Autodesk Inventor part; units mm, degrees
ref_plane "YZ Plane" through (0, 0, 0) normal (1, 0, 0) x (0, 1, 0)
ref_plane "XZ Plane" through (0, 0, 0) normal (0, 1, 0) x (-1, 0, 0)
ref_plane "XY Plane" through (0, 0, 0) normal (0, 0, 1) x (1, 0, 0)
sketch "Sketch1" plane through (0, 0, 0) normal (0, 1, 0) x (-1, 0, 0)
  line L0 (55, -86.5) -> (-55, -86.5)
  line L1 (-55, -86.5) -> (-55, 86.5)
  line L2 (-55, 86.5) -> (55, 86.5)
  line L3 (55, 86.5) -> (55, -86.5)
  line L4 (55, -86.5) -> (-55, 86.5) construction
  line L5 (-55, -86.5) -> (55, 86.5) construction
  point P0 (0, 0)
  dimension "d0" = 110
  dimension "d1" = 173
extrude "Extrusion1" add sketch "Sketch1" along normal blind 5
sketch "Sketch2" plane through (0, 5, 0) normal (0, 1, 0) x (1, 0, 0)
  line L0 (-55, -86.5) -> (55, -86.5)
  line L1 (-55, -86.5) -> (-60, -86.5)
  line L2 (-60, -86.5) -> (-60, 86.5)
  line L3 (-60, 86.5) -> (-55, 86.5)
  line L4 (-55, 86.5) -> (-55, -86.5)
  point P0 (0, 0)
  dimension "d4" = 5
extrude "Extrusion2" add sketch "Sketch2" against normal blind 34.5
sketch "Sketch3" plane through (0, 5, 0) normal (0, 1, 0) x (1, 0, 0)
  line L0 (55, -86.5) -> (55, 86.5)
  line L1 (55, -86.5) -> (60, -86.5)
  line L2 (60, -86.5) -> (60, 86.5)
  line L3 (60, 86.5) -> (55, 86.5)
  line L4 (55, 86.5) -> (55, -86.5)
  point P0 (0, 0)
  dimension "d7" = 5
extrude "Extrusion3" add sketch "Sketch3" against normal blind 34.5
sketch "Sketch4" plane through (-60, -29.5, 86.5) normal (0, 0, 1) x (1, 0, 0)
  line L0 (5, 29.5) -> (5, 0)
  line L1 (5, 29.5) -> (15, 29.5)
  line L2 (15, 29.5) -> (15, 19.5)
  line L3 (15, 19.5) -> (5, 19.5)
  line L4 (5, 19.5) -> (5, 29.5)
  circle A0 centre (10, 24.5) radius 3
  point P0 (60, 29.5)
  point P1 (5, 19.5)
  dimension "d10" = 10
  dimension "d11" = 10
  dimension "d23" = 5
  dimension "d24" = 5
  dimension "d26" = 6
extrude "Extrusion4" add sketch "Sketch4" against normal blind 5
pattern_linear "Rectangular Pattern1" count 2 spacing 100 along (1, 0, 0) count 2 spacing 168 along (0, 0, -1) of "Extrusion4"
fillet "Fillet3" radius 2 12 edges at (-55, -10, 84) (-45, -10, 84) (-45, 0, 84) (45, -10, 84) (55, -10, 84) (45, 0, 84) (45, -10, -84) (55, -10, -84) (45, 0, -84) (-55, -10, -84) (-45, -10, -84) (-45, 0, -84)
sketch "Sketch7" plane through (-60, 5, -86.5) normal (-1, 0, 0) x (0, 0, 1)
  line L0 (53, -16.5) -> (40, -16.5)
  line L1 (40, -16.5) -> (40, -25.5)
  line L2 (40, -25.5) -> (53, -25.5)
  line L3 (53, -25.5) -> (53, -16.5)
  line L4 (53, -16.5) -> (40, -25.5) construction
  line L5 (40, -16.5) -> (53, -25.5) construction
  line L6 (0, 0) -> (0, -34.5)
  line L7 (173, -34.5) -> (0, -34.5)
  point P0 (86.5, -5)
  point P1 (46.5, -21)
  dimension "d33" = 9
  dimension "d34" = 13
  dimension "d35" = 40
extrude "Extrusion6" cut sketch "Sketch7" against normal blind 5
sketch "Sketch8" plane through (0, 0, 0) normal (0, -1, 0) x (1, 0, 0)
  circle A0 centre (-50, 76.5) radius 1.25
  line L0 (-47, 81.5) -> (-53, 81.5)
  line L1 (-55, -86.5) -> (-55, 86.5)
  line L2 (-55, 71.5) -> (-45, 71.5)
  line L3 (-45, 71.5) -> (-45, 81.5)
  line L4 (-45, 81.5) -> (-55, 81.5)
  line L5 (-55, 81.5) -> (-55, 71.5)
  line L6 (-55, 71.5) -> (-45, 81.5) construction
  line L7 (-45, 71.5) -> (-55, 81.5) construction
  point P0 (0, 0)
  dimension "d39" = 2.5
  dimension "d40" = 5
  dimension "d41" = 5
  dimension "d42" = 10
  dimension "d43" = 10
extrude "Extrusion7" add sketch "Sketch8" along normal blind 19.5 contours A0 | L4 L3 L2 L1 L0
pattern_linear "Rectangular Pattern2" count 2 spacing 85.8 along (1, 0, 0) count 2 spacing 57.4 along (0, 0, -1) of "Extrusion7"
properties part number "Caja1"
The listing builds one solid part. Answer for the finished solid, in the listing's coordinates (mm). A direction names the side the tool comes from. Give positions to 0.01 mm unless a question says otherwise; leave off trailing zeros. Order: outer loops, then holes, each group sorted by start corner. A loop starts at its lowest first (then second) coordinate and runs counter-clockwise, first axis right, second up.
1) Find section C-C on y = -26.5. Write down the section's boundary in (x, z).
Reported:
outline: (-60, -86.5) - (-55, -86.5) - (-55, 86.5) - (-60, 86.5) - close; (55, -86.5) - (60, -86.5) - (60, 86.5) - (55, 86.5) - close
2) Find section B-B on x = -50. Write down the section's boundary in (y, z), then the cut area to 4 significant figures.
Reported:
outline: (-19.5, 14.1) - (0, 14.1) - (0, -81.5) - (-2, -81.5) - (-2, -86.5) - (5, -86.5) - (5, 86.5) - (-2, 86.5) - (-2, 81.5) - (-8, 81.5) - (-8, 86.5) - (-10, 86.5) - (-10, 81.5) - (-19.5, 81.5) - (-19.5, 71.5) - (0, 71.5) - (0, 24.1) - (-19.5, 24.1) - close; (-10, -86.5) - (-8, -86.5) - (-8, -81.5) - (-10, -81.5) - close
area: 1,295 mm2
3) Given P1, Ø5, axis at x = -48.5, y = -15.5, coming from the +Z side; P2, Ø2.5, axis at x = -50.5, z = -83.5, coming from the -Y side; P3, Ø5, axis at x = -50, y = -5, coming from the -Z side; P4, Ø2, axis at x = -43.5, y = -0.5, coming from the -Z side, each flat-ended and moving along its own axis, determine where each tip first touches the part or whether it passes through.
Reported:
P1: stops at z = 81.5
P2: stops at y = -10
P3: stops at z = 14.1
P4: stops at z = -86.5
4) Consider line 1 along X through (y, z) = (-1.5, 45); line 2 along Y through (x, z) = (50, -82.85); line 3 along Y through (x, z) = (-25.5, -74). Determine where each line is inside the solid, lowest interval first.
Reported:
line 1: x = -60 to -55, 55 to 60
line 2: y = -10 to -8, -2 to 5
line 3: y = 0 to 5
5) Find section A-A on x = 50. Write down the section's boundary in (y, z).
Reported:
outline: (-10, -86.5) - (-8, -86.5) - (-8, -81.5) - (-10, -81.5) - close; (-10, 81.5) - (-8, 81.5) - (-8, 86.5) - (-10, 86.5) - close; (-2, -86.5) - (5, -86.5) - (5, 86.5) - (-2, 86.5) - (-2, 81.5) - (0, 81.5) - (0, -81.5) - (-2, -81.5) - close
6) For faces 4 (the face through (36, -10, 14.1)), 5 (the face through (-50, -10, 84)), 6 (the face through (36, -10, 24.1)), 7 (the face through (50, -10, 84)), determine the directions among +Z, -Z, +X, -X, +Y, -Y from which every point of the face is accessible in a straight line to the end or side of a thin tool.
Reported:
face 4: -Z, -Y
face 5: +Z, -Y
face 6: -Y
face 7: +Z, -Z, -Y
7) Determine the mould class of faces 1 (the face through (-50, -10, 24.1)), 2 (the face through (-50, -5, 81.5)), 3 (the face through (-50, -10, -84)) for opening direction Y: pulls with the +Y half, pulls with the -Y half, needs draft (parallel to the pull), parting line crosses it, or undercut.
Reported:
face 1: needs draft
face 2: undercut
face 3: pulls with the -Y half
8) Find section D-D on z = 17.5. Write down the section's boundary in (x, y).
Reported:
outline: (-60, -29.5) - (-55, -29.5) - (-55, -19.5) - (-45, -19.5) - (-45, 0) - (30.8, 0) - (30.8, -19.5) - (40.8, -19.5) - (40.8, 0) - (55, 0) - (55, -29.5) - (60, -29.5) - (60, 5) - (-60, 5) - close
